Geometry check sheet. Reference: drawing and pictorial views, mm from the part's lowest x, y, z. Round coordinates to 2 decimals unless told otherwise and drop trailing zeros. Order: outer loops, then holes, each group sorted by start corner. A loop starts at its lowest first (then second) coordinate and runs counter-clockwise, first axis right, second up.
Q1. Cross-section at D-D on x = 14.5. Record the cut outline in (y, z).
Q2. Depth check by flat-ended pin: P1, Ø1.5, axis at y = 13, z = 24, coming from the +X side; P2, Ø12, axis at y = 53.5, z = 11.5, coming from the +X side; P3, Ø1.5, axis at y = 29, z = 53.5, coming from the -X side. Enter the tip coordinate at first touch or a pass-through.
Q3. Cross-section at A-A on y = 31. Record the cut outline in (x, z).
Q4. Mould release check, pull along Y, two halves, no side actions. Record for the marked faces 1, 2 and 3: +Y half, -Y half, draft (parallel to the pull), parting line (faces both ways), or undercut.
Q5. Cross-section at C-C on z = 29. Record the cut outline in (x, y).
Q6. Scan lines: probe 1 along Y at (x, z) = (31, 38); probe 2 along Y at (x, z) = (24, 42); probe 3 along X at (y, z) = (42.5, 36). Record each from-to range of solid material in increasing order.
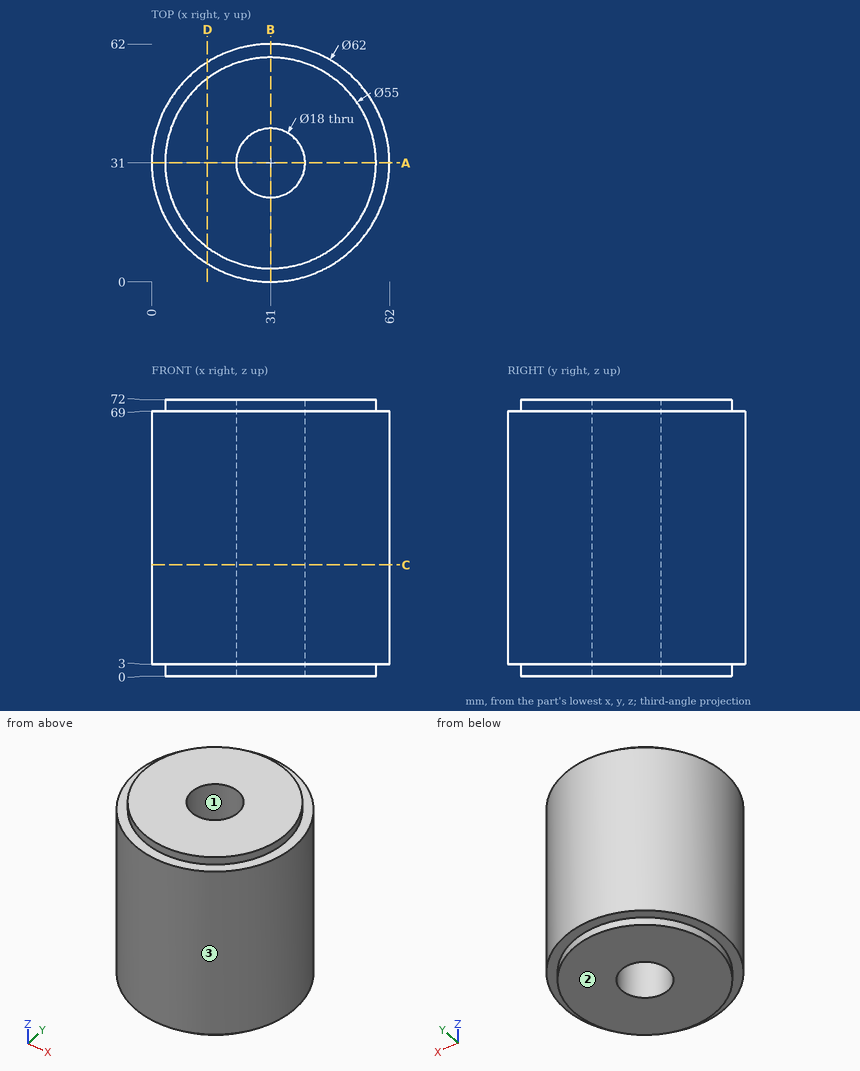
Results found:
1. outline: (4.76, 3) - (9, 3) - (9, 0) - (53, 0) - (53, 3) - (57.24, 3) - (57.24, 69) - (53, 69) - (53, 72) - (9, 72) - (9, 69) - (4.76, 69) - close
2. P1: stops at x = 56.76
2. P2: stops at x = 57.24
2. P3: stops at x = 0.03
3. outline: (0, 3) - (3.5, 3) - (3.5, 0) - (22, 0) - (22, 72) - (3.5, 72) - (3.5, 69) - (0, 69) - close; (40, 0) - (58.5, 0) - (58.5, 3) - (62, 3) - (62, 69) - (58.5, 69) - (58.5, 72) - (40, 72) - close
4. face 1: undercut
4. face 2: draft
4. face 3: parting line
5. outline: circle Ø62 at (31, 31); hole circle Ø18 at (31, 31)
6. probe 1: y = 0 to 22, 40 to 62
6. probe 2: y = 0.8 to 25.34, 36.66 to 61.2
6. probe 3: x = 2.21 to 59.79
